```python
from build123d import *

# Parameters (mm, degrees)
BOSS_EXTRUDE1_DEPTH      = 2
BOSS_EXTRUDE1_DEPTH_BACK = 2
SKETCH2_R                = 5
CIRPATTERN1_COUNT        = 6
SKETCH5_R                = 1
CUT_EXTRUDE1_DEPTH       = 3


with BuildPart() as part:
    # Sketch1 → Revolve1 (revolve)
    with BuildSketch(Plane.XY, mode=Mode.PRIVATE) as revolve1_sk:
        with BuildLine():
            Line((25.5, 1.5), (25.5, -1.5))
            ThreePointArc((25.5, -1.5), (25, -2), (24.5, -1.5))
            Line((24.5, -1.5), (24.5, 1.5))
            ThreePointArc((24.5, 1.5), (25, 2), (25.5, 1.5))
        make_face()
    revolve(revolve1_sk.sketch.rotate(Axis((0, 4.258241229, 0), (0, -1, 0)), 90), axis=Axis((0, 4.258241229, 0), (0, -1, 0)))



with BuildPart() as body_2:
    # Sketch2 → Boss-Extrude1 (new, two sides: drawn at the far end of the back side and taken through both)
    with BuildSketch(Plane(origin=(0, 0, 0), x_dir=(1, 0, 0), z_dir=(0, 1, 0)).offset(-BOSS_EXTRUDE1_DEPTH_BACK)):
        with Locations(Location((0, 0, 0), (0, 0, 270))):
            Circle(SKETCH2_R)
    extrude(amount=BOSS_EXTRUDE1_DEPTH + BOSS_EXTRUDE1_DEPTH_BACK)


with BuildPart() as part_1:
    add(part.part)

    add(body_2.part)  # Loft1 merges body 2
    # Sketch4 → Loft1 section 0
    with BuildSketch(Plane(origin=(25, 0, 0), x_dir=(0, 0, -1), z_dir=(1, 0, 0))):
        with BuildLine():
            Line((4.5, -1.5), (-4.5, -1.5))
            Line((-4.5, -1.5), (-4.5, 1.5))
            Line((-4.5, 1.5), (4.5, 1.5))
            Line((4.5, 1.5), (4.5, -1.5))
        make_face()
    # Sketch3 → Loft1 section 1
    with BuildSketch(Plane(origin=(4, 0, 0), x_dir=(0, 0, -1), z_dir=(1, 0, 0))):
        with BuildLine():
            Line((2.25, -0.75), (-2.25, -0.75))
            Line((-2.25, -0.75), (-2.25, 0.75))
            Line((-2.25, 0.75), (2.25, 0.75))
            Line((2.25, 0.75), (2.25, -0.75))
        make_face()
    loft1 = loft()

    # CirPattern1: Loft1 ×6 about axis
    cirpattern1_axis = Axis((0, 0, 0), (0, 1, 0))
    for i in range(1, CIRPATTERN1_COUNT):
        add(loft1.rotate(cirpattern1_axis, i * 360 / CIRPATTERN1_COUNT))

    # Sketch5 → Cut-Extrude1 (cut)
    with BuildSketch(Plane(origin=(0, 2, 0), x_dir=(1, 0, 0), z_dir=(0, 1, 0))):
        with Locations(Location((0, 0, 0), (0, 0, 270))):
            Circle(SKETCH5_R)
    extrude(amount=-CUT_EXTRUDE1_DEPTH, mode=Mode.SUBTRACT)


solid = part_1.part
```
Read the model definition and answer for the solid it produces. Units are mm, in the model's axes. A direction names the side the tool comes from. Coordinates: 2 decimals unless noted, no trailing zeros. Answer as a JSON object with one key per item and string values. Group by question number.
1. Each of these flat-tipped pins is pushed along its axis until it touches: P1, Ø8, axis at x = -10, z = 12.5, coming from the +Y side; P2, Ø1.6, axis at x = 0.5, z = -0.5, coming from the +Y side; P3, Ø4, axis at x = 5.5, z = 4.5, coming from the +Y side; P4, Ø3, axis at x = -7.5, z = 9.5, coming from the -Y side. Where does it stop, or does it pass through?
2. A cutting plane is placed at A-A (x = 12). Give the number of separate pieces and of enclosed holes in the cut face, plus the area to 3 significant figures.
3. Consider L1, parallel to X at y = 0, z = 0; L2, parallel to X at y = -0.15, z = -6; L3, parallel to Z at x = 20.5, y = 0.25. Determine where each line is inside the solid, lowest interval first. Write a range as [from, to].
4. Which of the six approach directions +Z, -Z, +X, -X, +Y, -Y give full straight-line access (tool end or side, diameter ignored) to faces 1 (the flat face through (0, -2, 0)), 2 (the cylindrical face through (0, 0, -5)), 3 (the flat face through (0, -1, 0))?
5. The mould has two halves that part along Z. Classify faces 4 (the cylindrical face through (-7.36, 0.02, 23.37)), 5 (the flat face through (1.2, 2, -0.1)), 6 (the cylindrical face through (15.516, -0.021, -20.236)): +Z half, -Z half, draft (parallel to the pull), parting line (faces both ways), or undercut.
Worked out:
{
 "1": {"P1": "stops at y = 1.32", "P2": "stops at y = 2", "P3": "stops at y = 0.92", "P4": "stops at y = -1.09"},
 "2": {"separate pieces": "3", "enclosed holes": "0", "area": "64.9 mm²"},
 "3": {"L1": "x = [-25.5, -1], [1, 25.5]", "L2": "x = [-24.78, -23.75], [-6.62, -0.68], [0.68, 6.62], [23.75, 24.78]", "L3": "z = [-15.17, -13.42], [-4.02, 4.02], [13.42, 15.17]"},
 "4": {"face 1": "+Z, -Z, +X, -X, -Y", "face 2": "none", "face 3": "+Y"},
 "5": {"face 4": "undercut", "face 5": "draft", "face 6": "parting line"}
}
